Check sheet for the modelled part. Datum: model origin and axes. Units: mm. Coordinates: 2 decimals unless noted, no trailing zeros. Order: outer loops, then holes, each group sorted by start corner. A loop starts at its lowest first (then second) coordinate and runs counter-clockwise, first axis right, second up.
from build123d import *

# Parameters (mm, degrees)
SKETCH_1_R          = 12.5
SKETCH_1_R_2        = 11.5
EXTRUDE_1_DEPTH     = 201.7
SKETCH_3_R          = 2.5
CUT_EXTRUDE_1_DEPTH = 50


with BuildPart() as part:
    # 草图1 → 凸台-拉伸1 (new, symmetric)
    with BuildSketch(Plane.XY):
        Circle(SKETCH_1_R)
        Circle(SKETCH_1_R_2, mode=Mode.SUBTRACT)
    extrude(amount=EXTRUDE_1_DEPTH, both=True)

    # 草图3 → 切除-拉伸1 (cut, symmetric)
    with BuildSketch(Plane(origin=(0, 0, 0), x_dir=(1, 0, 0), z_dir=(0, 1, 0))):
        with Locations(Location((0, 67.5, 0), (0, 0, 270))):
            Circle(SKETCH_3_R)
        with Locations(Location((0, -67.5, 0), (0, 0, 270))):
            Circle(SKETCH_3_R)
    extrude(amount=CUT_EXTRUDE_1_DEPTH, both=True, mode=Mode.SUBTRACT)


solid = part.part
(1) Thickness scan on probe 1 along Z at (x, y) = (0, 11.9); probe 2 along Y at (x, z) = (-1.25, -41.5); probe 3 along Y at (x, z) = (-0.25, 95). Record the ranges inside material, lowest first.
Filled in:
probe 1: z = -201.7 to -70, -65 to 65, 70 to 201.7
probe 2: y = -12.44 to -11.43, 11.43 to 12.44
probe 3: y = -12.5 to -11.5, 11.5 to 12.5
(2) Go/stop test with flat-tipped pins: P1, Ø4, axis at x = 0, z = -67.5, coming from the +Y side; P2, Ø3, axis at x = -3.5, z = -143, coming from the +Y side; P3, Ø4, axis at x = -2.5, z = -19, coming from the +Y side; P4, Ø5, axis at x = 3.5, z = -125, coming from the -Y side. Record where each tip stops, or that it passes through.
Filled in:
P1: passes through
P2: stops at y = 12.34
P3: stops at y = 12.49
P4: stops at y = -12.46
(3) Cross-section at A-A (y = 0). Enter the section's corners in (x, z), and give its area (3 significant figures).
Filled in:
outline: (-12.5, -201.7) - (-11.5, -201.7) - (-11.5, 201.7) - (-12.5, 201.7) - close; (11.5, -201.7) - (12.5, -201.7) - (12.5, 201.7) - (11.5, 201.7) - close
area: 807 mm2
(4) Cross-section at B-B (x = -8). Enter the section's corners in (y, z), and give its area (3 significant figures).
Filled in:
outline: (-9.6, -201.7) - (-8.26, -201.7) - (-8.26, 201.7) - (-9.6, 201.7) - close; (8.26, -201.7) - (9.6, -201.7) - (9.6, 201.7) - (8.26, 201.7) - close
area: 1,080 mm2
(5) Cross-section at C-C (z = 118.5). Enter the section's corners in (x, y), and give its area (3 significant figures).
Filled in:
outline: circle Ø25 at (0, 0); hole circle Ø23 at (0, 0)
area: 75.4 mm2
